```python
from build123d import *

# Parameters (mm, degrees)
SKETCH_1_R      = 1.5
EXTRUDE_1_DEPTH = 1.5
SKETCH_4_R      = 3
SKETCH_4_R_2    = 1.5
EXTRUDE_2_DEPTH = 6
FILLET_1_R      = 1


with BuildPart() as part:
    # Эскиз1 → Бобышка-Вытянуть1 (new body)
    with BuildSketch(Plane.XY):
        with BuildLine():
            ThreePointArc((-14.696938457, 3), (-14.848853857, -2.124038405), (-13.266499161, -7))
            Line((-13.266499161, -7), (13.266499161, -7))
            ThreePointArc((13.266499161, -7), (14.848853857, -2.124038405), (14.696938457, 3))
            Line((14.696938457, 3), (27.493638863, 8.666206601))
            ThreePointArc((27.493638863, 8.666206601), (29.425159504, 15.327651899), (22.841677521, 17.51017118))
            ThreePointArc((22.841677521, 17.51017118), (21.287556094, 16.919662188), (19.657078674, 16.594796577))
            Line((19.657078674, 16.594796577), (3, 14.696938457))
            Line((3, 14.696938457), (-3, 14.696938457))
            Line((-3, 14.696938457), (-19.657078674, 16.594796577))
            ThreePointArc((-19.657078674, 16.594796577), (-21.287556094, 16.919662188), (-22.841677521, 17.51017118))
            ThreePointArc((-22.841677521, 17.51017118), (-29.543661072, 15.086898192), (-27.014954435, 8.423980045))
            Line((-27.014954435, 8.423980045), (-14.696938457, 3))
        make_face()
        with Locations((-25, 13)):
            Circle(SKETCH_1_R, mode=Mode.SUBTRACT)
        with Locations((25, 13)):
            Circle(SKETCH_1_R, mode=Mode.SUBTRACT)
    extrude(amount=EXTRUDE_1_DEPTH)

    # Эскиз4 → Бобышка-Вытянуть2 (add)
    with BuildSketch(Plane(origin=(0, 0, 0), x_dir=(-1, 0, 0), z_dir=(0, 0, -1))):
        with Locations((25, 13)):
            Circle(SKETCH_4_R)
        with Locations((25, 13)):
            Circle(SKETCH_4_R_2, mode=Mode.SUBTRACT)
        with Locations((-25, 13)):
            Circle(SKETCH_4_R)
        with Locations((-25, 13)):
            Circle(SKETCH_4_R_2, mode=Mode.SUBTRACT)
    extrude(amount=EXTRUDE_2_DEPTH)

    # Скругление1
    fillet_1_edges = [part.edges().sort_by_distance(p)[0] for p in [
        (-22, 13, 0),
        (28, 13, 0),
    ]]
    fillet(fillet_1_edges, radius=FILLET_1_R)


solid = part.part
```
Geometry check sheet. Reference: the model listing, model coordinates, mm. A direction names the side the tool comes from. Round coordinates to 2 decimals unless told otherwise and drop trailing zeros. Order: outer loops, then holes, each group sorted by start corner. A loop starts at its lowest first (then second) coordinate and runs counter-clockwise, first axis right, second up. Notation, with made-up numbers: M 77.5,61 L 116.5,61 A8 ccw 116.5,71 Z; hole C 10.5,43 d11. An arc over 180 degrees is marked long. Answer as CSV lines item,"result".
1) Sectioned sample at A-A on y = 13. Record the cut outline in (x, z), and give its area (3 significant figures).
Entries:
outline,"M -30,0 L -29,0 A1 cw -28,-1 L -28,-6 L -26.5,-6 L -26.5,1.5 L -30,1.5 Z; M -23.5,-6 L -22,-6 L -22,-1 A1 cw -21,0 L 21,0 A1 cw 22,-1 L 22,-6 L 23.5,-6 L 23.5,1.5 L -23.5,1.5 Z; M 26.5,-6 L 28,-6 L 28,-1 A1 cw 29,0 L 30,0 L 30,1.5 L 26.5,1.5 Z"
area,"118 mm2"
2) Sectioned sample at B-B on x = 25. Record the cut outline in (y, z), and give its area (3 significant figures).
Entries:
outline,"M 7.56,0 L 9,0 A1 cw 10,-1 L 10,-6 L 11.5,-6 L 11.5,1.5 L 7.56,1.5 Z; M 14.5,-6 L 16,-6 L 16,-1 A1 cw 17,0 L 18,0 L 18,1.5 L 14.5,1.5 Z"
area,"29.6 mm2"
3) Gauge pin test, flat ends, axial feed: pin 1 Ø10 at (x, y) = (23.5, -1) entering from +Z; pin 2 Ø1.5 at (y, z) = (-1.5, 0) entering from +X; pin 3 Ø8 at (x, y) = (0, 15.5) entering from -Z; pin 4 Ø0.8 at (x, z) = (0.5, 1) entering from +Y. Record the tip position at first contact, or that the pin passes through.
Entries:
pin 1,"through"
pin 2,"x = 14.98"
pin 3,"z = 0"
pin 4,"y = 14.7"
4) Thickness scan on probe 1 along Z at (x, y) = (-3, -4.5); probe 2 along Y at (x, z) = (-25, 1.25); probe 3 along Y at (x, z) = (25, 0.9). Record the ranges inside material, lowest first. Write a range as [from, to].
Entries:
probe 1,"[0, 1.5]"
probe 2,"[7.54, 11.5], [14.5, 18]"
probe 3,"[7.56, 11.5], [14.5, 18]"
5) Mould release check, pull along X, two halves, no side actions. Record for faces 1 (the face through (21.006, 5.793, 0.74)), 2 (the face through (-14.86, -2.05, 0.74)), 3 (the face through (0, 6, 1.5)), 4 (the face through (-24.35, 10.07, -3.46)): +X half, -X half, draft (parallel to the pull), parting line (faces both ways), or undercut.
Entries:
face 1,"+X half"
face 2,"-X half"
face 3,"draft"
face 4,"undercut"
6) Sectioned sample at D-D on x = 1.5. Record the cut outline in (y, z), and give its area (3 significant figures).
Entries:
outline,"M -7,0 L 14.7,0 L 14.7,1.5 L -7,1.5 Z"
area,"32.5 mm2"
7) Tool access check on faces 5 (the face through (14.838, -2.195, 0.74)), 6 (the face through (-21.265, 16.913, 0.74)), 7 (the face through (27.4, 11.2, -3.5)). Record the directions out of +Z, -Z, +X, -X, +Y, -Y that give a thin tool (end or side, any length) a straight path to the whole face; none if there is none.
Entries:
face 5,"+Z, -Z, +X"
face 6,"+Z, -Z, +Y"
face 7,"-Z"
8) Sectioned sample at C-C on z = -5. Record the cut outline in (x, y).
Entries:
outline,"C -25,13 d6; C 25,13 d6; hole C -25,13 d3; hole C 25,13 d3"
